Answer from the drawing. Dimensions are ordinates in mm from the lowest x, y and z of the part. Coordinates: 2 decimals unless noted, no trailing zeros. Write each loop counter-clockwise with the first axis right and the second up, starting at its lowest first coordinate (ties: lowest second). Pieces come first, ordered by that corner, then holes. Notation, with made-up numbers: (-27.75, 31) - (-4.75, 31) arc R28 cw to (-4.75, 53) - close; hole circle Ø3 at (34, 23). An arc over 180 degrees is marked (long way). Use one line per item in the form item = value. Start each with the question number.
Item 1: Determine the mould class of the marked faces 1, 2 and 3 for opening direction Z: released by +Z, released by -Z, zero draft, split by the parting line, or undercut.
Item 2: A cutting plane is placed at D-D (z = 25). Write down the section's boundary in (x, y).
Item 3: Given pin 1 (1.7 mm diameter, centred on x = 15.5, z = 61.5, fed in from -Y); pin 2 (7.5 mm diameter, centred on x = 71.44, z = 38.1, fed in from -Y); pin 3 (3 mm diameter, centred on x = 63, y = 4.5, fed in from -Z); pin 4 (1 mm diameter, centred on x = 8, y = 2.5, fed in from +Z), each flat-ended and moving along its own axis, determine where each tip first touches the part or whether it passes through.
Item 4: Consider probe 1 along X at (y, z) = (0.8, 38.1) (1 decimal); probe 2 along X at (y, z) = (4.2, 38.1) (1 decimal); probe 3 along Z at (x, y) = (38, 4). Determine where each line is inside the solid, lowest interval first.
Item 5: A cutting plane is placed at A-A (x = 38.1). Give the number of separate pieces and of enclosed holes in the cut face.
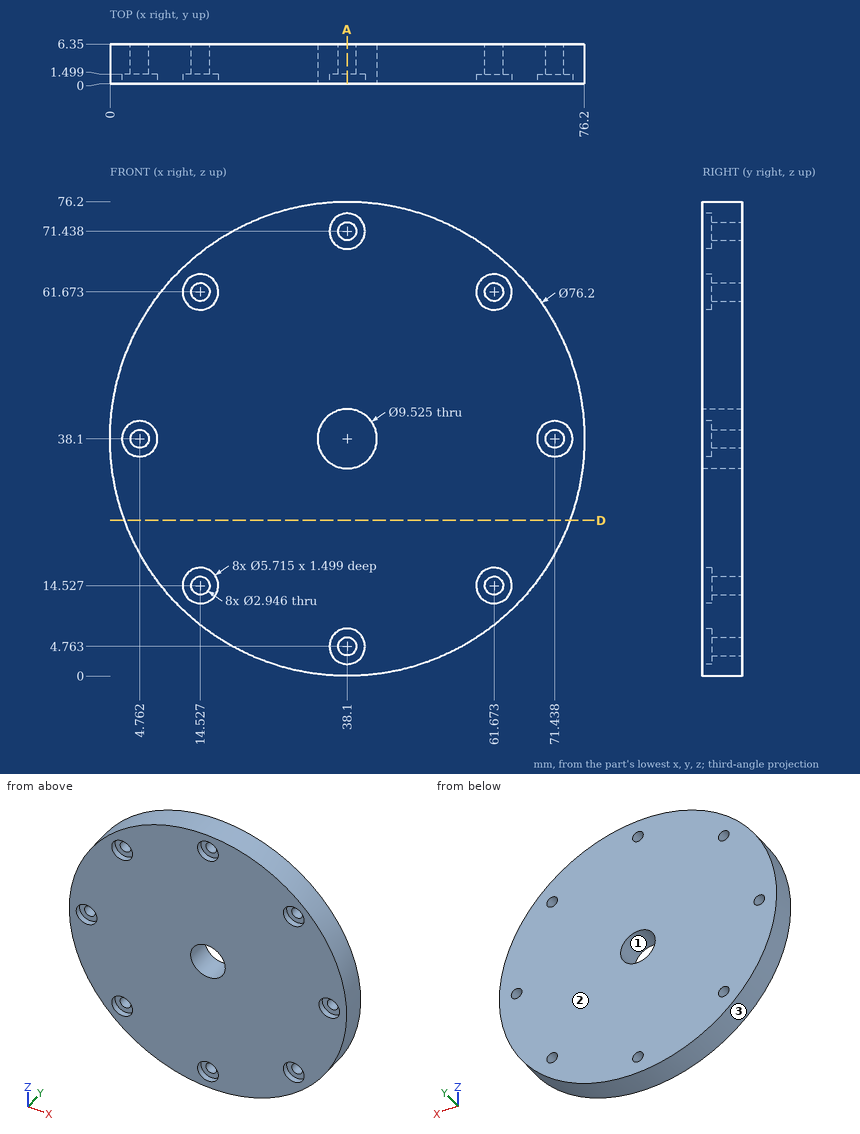
Answer:
q1.face_1 = undercut
q1.face_2 = zero draft
q1.face_3 = split by the parting line
q2.outline = (2.32, 0) - (73.88, 0) - (73.88, 6.35) - (2.32, 6.35) - close
q3.pin_1 = 1.5
q3.pin_2 = 0
q3.pin_3 = 8.03
q3.pin_4 = 62.09
q4.probe_1 = 0 to 1.9, 7.6 to 33.3, 42.9 to 68.6, 74.3 to 76.2
q4.probe_2 = 0 to 3.3, 6.2 to 33.3, 42.9 to 70, 72.9 to 76.2
q4.probe_3 = 0 to 3.29, 6.23 to 33.34, 42.86 to 69.97, 72.91 to 76.2
q5.separate_pieces = 4
q5.enclosed_holes = 0
